Work out the finished part from the listing and answer in its coordinate system (mm). Give positions to 0.01 mm unless a question says otherwise; leave off trailing zeros. Loops run counter-clockwise (first coordinate to the right, second up) from the corner with the lowest first, then second, coordinate; pieces in that order, holes last. Notation, with made-up numbers: (24, -9.5) - (31, -9.5) arc R20 cw to (31, 19.5) - close; hole circle Ø7 at (66.5, 58.5). An arc over 180 degrees is marked (long way). One line per question, with ' | ' between items. Start each with the question number.
1. Each of these flat-tipped pins is pushed along its axis until it touches: pin 1 (5 mm diameter, centred on x = 9, y = -6, fed in from +Z); pin 2 (3 mm diameter, centred on y = -3.5, z = -18.5, fed in from +X). Where does it stop, or does it pass through?
2. Section C-C (z = -70.5) is taken. Determine the outline of the cut face in (x, y), plus the area to 3 significant figures.
3. Find the intervals of material crossed by line 1 (Z direction, x = 94, y = -19); line 2 (Z direction, x = -12, y = -15.5); line 3 (X direction, y = -7, z = -101), in increasing order.
4. Section B-B (y = -7.5) is taken. Determine the outline of the cut face in (x, z).
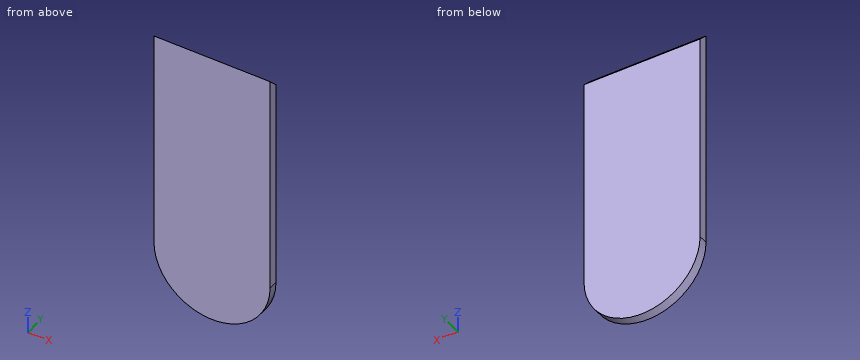
from build123d import *

# Parameters (mm, degrees)
F1_DEPTH = 20
F0_W     = 250
F0_H     = 475
F2_DEPTH = 20
F3_SIZE  = 19.99999


# Not quite as in the source:
# - a fillet or chamfer is up to 0.001 mm smaller than in the source, because OpenCascade refuses the exact size


with BuildPart() as f1:
    # F0 (on Front) → F1 (new body)
    with BuildSketch(Plane.XZ):
        with BuildLine():
            Line((123.788267374, 0), (-126.211732626, 0))
            ThreePointArc((-126.211732626, 0), (-1.211732626, -125), (123.788267374, 0))
        make_face()
    extrude(amount=F1_DEPTH)

    # F0 (on Front) → F2 (join)
    with BuildSketch(Plane.XZ):
        with Locations((-1.211732626, 237.5)):
            Rectangle(F0_W, F0_H)
    extrude(amount=F2_DEPTH)

    # F3 (size 20 in the source; OpenCascade refuses exactly that, so slightly less here)
    f3_edges = [f1.edges().sort_by_distance(p)[0] for p in [
        (-1.211733, 0, 475),
    ]]
    chamfer(f3_edges, length=F3_SIZE)


solid = f1.part
Conclusion:
1) pin 1: z = 463.5 | pin 2: x = 122.63
2) outline: (-104.43, -20) - (102.01, -20) - (102.01, 0) - (-104.43, 0) - close | area: 4,130 mm²
3) line 1: -80.99 to 474 | line 2: -124.53 to 470.5 | line 3: -74.86 to 72.44
4) outline: (-126.21, 0) arc R125 ccw to (123.79, 0) - (123.79, 462.5) - (-126.21, 462.5) - close
